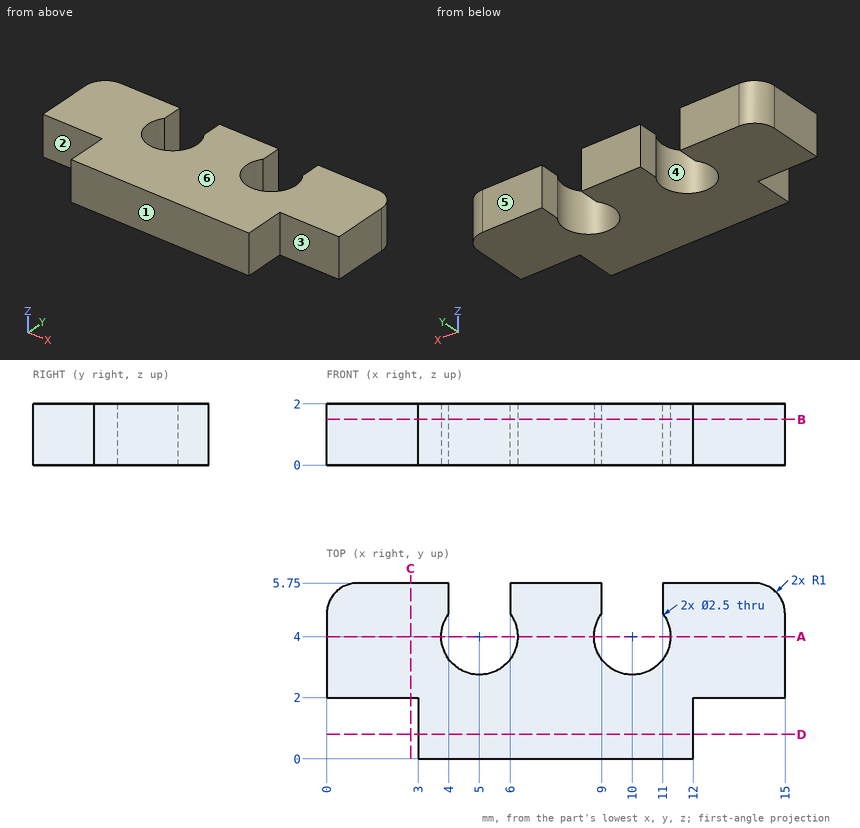
Here's the drawing with two shaded views (mm, measured from the low corner). I have some questions. A direction names the side the tool comes from. Coordinates: 2 decimals unless noted, no trailing zeros. Order: outer loops, then holes, each group sorted by start corner. A loop starts at its lowest first (then second) coordinate and runs counter-clockwise, first axis right, second up. Notation, with made-up numbers: (-9.75, 86) - (1.25, 86) arc R11 ccw to (1.25, 95) - close; hole circle Ø7 at (26, 20.5). An arc over 180 degrees is marked (long way). Answer in a Markdown table with one row per item. Add a question column.
(1) Will these pins go through, and if not, where does the flat tip stop? pin 1 (0.8 mm diameter, centred on y = 5.5, z = 1, fed in from +X); pin 2 (0.5 mm diameter, centred on y = 5.5, z = 1, fed in from -X); pin 3 (2 mm diameter, centred on x = 5, y = 4, fed in from -Z); pin 4 (0.6 mm diameter, centred on y = 1, z = 1.5, fed in from -X).
(2) If we section it at D-D, the plane y = 0.8: Please give me the cut outline in (x, z), then the cut area to 3 significant figures.
(3) I need wall thicknesses on L1, parallel to X at y = 4.1, z = 1.05; L2, parallel to X at y = 5.5, z = 0.6; L3, parallel to X at y = 0.3, z = 1.7. Which ranges of each line are inside material? Lowest first, please.
(4) If we section it at C-C, the plane x = 2.75: Please give me the cut outline in (y, z), then the cut area to 3 significant figures.
(5) On a 3-axis mill with a long thin cutter (end or side, diameter ignored), from which of +Z, -Z, +X, -X, +Y, -Y can I reach the whole of each face in a straight line? I mean the marked faces 1, 2 and 3. Say none if no direction works.
(6) If we section it at B-B, the plane z = 1.5: Please give me the cut outline in (x, y).
(7) If we section it at A-A, the plane y = 4: Please give me the cut outline in (x, z).
(8) If we mould it in two halves opening along Y, with no side actions, what happens to the marked faces 4, 5 and 6? For each: released by +Y, released by -Y, zero draft, split by the parting line, or undercut.
Results are:
| question | item | result |
|---|---|---|
| 1 | pin 1 | stops at x = 14.94 |
| 1 | pin 2 | stops at x = 0.13 |
| 1 | pin 3 | passes through |
| 1 | pin 4 | stops at x = 3 |
| 2 | outline | (3, 0) - (12, 0) - (12, 2) - (3, 2) - close |
| 2 | area | 18.0 mm2 |
| 3 | L1 | x = 0 to 3.75, 6.25 to 8.75, 11.25 to 15 |
| 3 | L2 | x = 0.34 to 4, 6 to 9, 11 to 14.66 |
| 3 | L3 | x = 3 to 12 |
| 4 | outline | (2, 0) - (5.75, 0) - (5.75, 2) - (2, 2) - close |
| 4 | area | 7.50 mm2 |
| 5 | face 1 | +Z, -Z, +X, -X, -Y |
| 5 | face 2 | +Z, -Z, -X, -Y |
| 5 | face 3 | +Z, -Z, +X, -Y |
| 6 | outline | (0, 2) - (3, 2) - (3, 0) - (12, 0) - (12, 2) - (15, 2) - (15, 4.75) arc R1 ccw to (14, 5.75) - (11, 5.75) - (11, 4.75) arc R1.25 cw (long way) to (9, 4.75) - (9, 5.75) - (6, 5.75) - (6, 4.75) arc R1.25 cw (long way) to (4, 4.75) - (4, 5.75) - (1, 5.75) arc R1 ccw to (0, 4.75) - close |
| 7 | outline | (0, 0) - (3.75, 0) - (3.75, 2) - (0, 2) - close; (6.25, 0) - (8.75, 0) - (8.75, 2) - (6.25, 2) - close; (11.25, 0) - (15, 0) - (15, 2) - (11.25, 2) - close |
| 8 | face 4 | undercut |
| 8 | face 5 | released by +Y |
| 8 | face 6 | zero draft |
